Autodesk Inventor part; units mm, degrees
ref_plane "YZ Plane" through (0, 0, 0) normal (1, 0, 0) x (0, 1, 0)
ref_plane "XZ Plane" through (0, 0, 0) normal (0, 1, 0) x (-1, 0, 0)
ref_plane "XY Plane" through (0, 0, 0) normal (0, 0, 1) x (1, 0, 0)
sketch "草图1" plane through (0, 0, 0) normal (0, 0, 1) x (1, 0, 0)
  arc A0 (19, 0) -> (0, 35.6791) centre (-24, 0) ccw
  line L0 (96, 34) -> (96, 0)
  line L1 (96, 34) -> (0, 42.3989)
  line L2 (-101.2978, 0) -> (181.6605, 0)
  line L3 (0, 42.3989) -> (0, 35.6791)
  point P0 (0, 0)
  dimension "d0" = 24
  dimension "d1" = 86
  dimension "d2" = 34
  dimension "d4" = 5
revolve "旋转1" add sketch "草图1" angle 360 about axis through (-101.2978, 0, 0) along (1, 0, 0)
sketch "草图2" plane through (96, 0, 0) normal (1, 0, 0) x (0, 0, -1)
  circle A0 centre (0, 0) radius 34
  point P0 (0, 0)
hole "孔1" at (96, 0, 0) direction (-1, 0, 0) diameter 36 depth 60
sketch "草图3" plane through (0, 0, 0) normal (0, 1, 0) x (-1, 0, 0)
  circle A0 centre (-56.72, 0) radius 12
  line L0 (-96, 34) -> (-96, -34)
  point P0 (0, 0)
  dimension "d13" = 24
  dimension "d14" = 39.28
extrude "拉伸1" cut sketch "草图3" along normal up to surface
sketch "草图4" plane through (0, 0, 0) normal (0, 0, 1) x (1, 0, 0)
  line L0 (96, 18) -> (96, -18)
  line L1 (36, -18) -> (36, 18)
  circle A0 centre (57.0565, 0) radius 12
  point P0 (0, 0)
  point P1 (56.72, 13.4164)
  point P2 (56.72, 13.4164)
  point P3 (57.0565, 35.4317)
  dimension "d17" = 24
extrude "拉伸2" cut sketch "草图4" against normal up to surface
properties part number "旋塞" material "不锈钢"
For this review, take the finished solid that the model builds, in its own axes (mm). A direction names the side the tool comes from. Give positions to 0.01 mm unless a question says otherwise; leave off trailing zeros. Order: outer loops, then holes, each group sorted by start corner. A loop starts at its lowest first (then second) coordinate and runs counter-clockwise, first axis right, second up. Notation, with made-up numbers: M 15.25,8.25 L 59.25,8.25 A21 cw 59.25,19.25 Z; hole C 84.5,-0.75 d4. An arc over 180 degrees is marked long. Answer in a Markdown table with one row per item. Add a question column.
(1) Mouldability with a two-part tool opening along X and no side actions: class faces 1 (the face through (45.635, 25.775, 4.596)), 2 (the face through (0, -19, -31)), 3 (the face through (96, 15, -15)) as +X half, -X half, draft (parallel to the pull), parting line (faces both ways), or undercut.
(2) Consider section B-B on x = 39. State the section outline as (y, z) points, and give its area (3 significant figures).
(3) Wall thickness on probe 1 along Z at (x, y) = (56, 26); probe 2 along Z at (x, y) = (80.5, 16.5); probe 3 along X at (y, z) = (32, 3.5): over which ranges is each line inside the solid? List them lowest first. Write a range as [from, to].
(4) For faces 4 (the face through (47.53, -7.3, -25.76)), 5 (the face through (36, 0, 0)), list the 3-axis set-ups (+Z, -Z, +X, -X, +Y, -Y) from which the entire face can be reached by the end or side of a thin tool; tool diameter is ignored.
(5) Consider section A-A on x = 56.72. State the section outline as (y, z) points, and give its area (3 significant figures).
(6) For pin 1 (11 mm diameter, centred on y = -4, z = 7, fed in from +X); pin 2 (1.5 mm diameter, centred on x = 29, y = -7, fed in from +Z); pin 3 (12 mm diameter, centred on x = 42.5, z = -24, fed in from -Y), all flat-tipped, find the tip position at first contact; note any pin that passes through.
(7) Consider section C-C on x = 76.5. State the section outline as (y, z) points, and give its area (3 significant figures).
Evaluation:
| question | item | result |
|---|---|---|
| 1 | face 1 | undercut |
| 1 | face 2 | -X half |
| 1 | face 3 | +X half |
| 2 | outline | C 0,0 d77.97; hole C 0,0 d36 |
| 2 | area | 3,760 mm^2 |
| 3 | probe 1 | z = [-27.02, -11.98], [11.98, 27.02] |
| 3 | probe 2 | z = [-31.27, -7.19], [7.19, 31.27] |
| 3 | probe 3 | x = [4.51, 45.24], [68.2, 96] |
| 4 | face 4 | -Z |
| 4 | face 5 | +X |
| 5 | outline | M -12,-35.46 L -12,-13.42 A18 cw long 13.42,12 L 35.46,12 A37.44 ccw long Z; M 12,-35.46 A37.44 ccw 35.46,-12 L 13.42,-12 A18 cw 12,-13.42 Z |
| 5 | area | 2,410 mm^2 |
| 6 | pin 1 | stops at x = 36 |
| 6 | pin 2 | stops at z = 39.39 |
| 6 | pin 3 | stops at y = -34.29 |
| 7 | outline | C 0,0 d71.41; hole C 0,0 d36 |
| 7 | area | 2,990 mm^2 |
